Can you work these out from the model? Positions are in its coordinate system, mm. A direction names the side the tool comes from. Give positions to 0.01 mm unless a question says otherwise; leave off trailing zeros. Write each loop counter-clockwise with the first axis right and the second up, starting at its lowest first coordinate (ties: lowest second). Pieces come first, ordered by that corner, then holes. Notation, with made-up numbers: M 75,-26.5 L 121,-26.5 A30 ccw 121,10.5 Z; hole C -32,4 d11. An arc over 180 degrees is marked long. Write each question's results on one line, items separated by ' | '.
from build123d import *

# Parameters (mm, degrees)
SALIENTE_EXTRUIR1_DEPTH = 6.9


with BuildPart() as part:
    # Croquis1 → Saliente-Extruir1 (new body)
    with BuildSketch(Plane.XY):
        with BuildLine():
            Line((-74.243930555, 54.648970741), (-34.403574409, -7.603291729))
            Line((-34.403574409, -7.603291729), (-43.204784385, -7.603291729))
            Line((-43.204784385, -7.603291729), (-80.487794166, 50.653007541))
            ThreePointArc((-80.487794166, 50.653007541), (-79.363843961, 55.772920947), (-74.243930555, 54.648970741))
        make_face()
        with BuildLine():
            Line((-79.629068495, 51.202576909), (-79.221671544, 53.058386092))
            ThreePointArc((-79.221671544, 53.058386092), (-75.765533956, 53.675171252), (-77.773259312, 50.795179958))
            Line((-77.773259312, 50.795179958), (-79.629068495, 51.202576909))
        make_face(mode=Mode.SUBTRACT)
    extrude(amount=SALIENTE_EXTRUIR1_DEPTH)


solid = part.part
Item 1: If I drill on line 1 (Y direction, x = -59, z = 6.25); line 2 (Y direction, x = -51, z = 3); line 3 (X direction, y = 52.5, z = 2.25), over which ranges is the centre line in solid material (lowest first)? Write a range as from..to.
Geometry says:
line 1: y = 17.08..30.83 | line 2: y = 4.58..18.33 | line 3: x = -81.07..-79.34, -75.47..-72.87
Item 2: I'm going to push flat-ended pins straight in: pin 1 (1 mm diameter, centred on x = -45, y = 12.5, fed in from -Z); pin 2 (3 mm diameter, centred on x = -52, z = 4.5, fed in from +Y); pin 3 (4 mm diameter, centred on y = 45.5, z = 5, fed in from +X). Where does each tip first touch, or does it pass through?
Geometry says:
pin 1: passes through | pin 2: stops at y = 22.24 | pin 3: stops at x = -67.11
Item 3: I want a section at D-D, the plane x = -51. Please give me the cut outline in (y, z), and give its area (3 significant figures).
Geometry says:
outline: M 4.58,0 L 18.33,0 L 18.33,6.9 L 4.58,6.9 Z | area: 94.9 mm2
Item 4: Thinking about a two-plate mould opening in X: for faces 3 (the face through (-39, -7.603, 3)), 4 (the face through (-75.8, 53.73, 3.4)), 5 (the face through (-54.603, 23.959, 3.402)), which applies, +X half, -X half, draft (parallel to the pull), parting line (faces both ways), or undercut?
Geometry says:
face 3: draft | face 4: undercut | face 5: +X half
Item 5: I want a section at A-A, the plane z = 4.75. Please give me the cut outline in (x, y).
Geometry says:
outline: M -80.49,50.65 L -43.2,-7.6 L -34.4,-7.6 L -74.24,54.65 A3.71 ccw Z; hole M -79.63,51.2 L -77.77,50.8 A1.9 ccw long -79.22,53.06 Z
Item 6: I want a section at B-B, the plane x = -77. Please give me the cut outline in (y, z).
Geometry says:
outline: M 45.2,0 L 50.79,0 L 50.79,6.9 L 45.2,6.9 Z; M 54.52,0 L 56.34,0 L 56.34,6.9 L 54.52,6.9 Z
Item 7: I want a section at C-C, the plane y = 0. Please give me the cut outline in (x, z).
Geometry says:
outline: M -48.07,0 L -39.27,0 L -39.27,6.9 L -48.07,6.9 Z
Item 8: For faces 1 (the face through (-58, 22, 0)), 2 (the face through (-78.7, 51, 3.4)), which set-ups out of +Z, -Z, +X, -X, +Y, -Y let a thin tool reach every point of the face, with its end or its side?
Geometry says:
face 1: -Z, +X, -X, +Y, -Y | face 2: +Z, -Z
